Check sheet for the modelled part. Datum: model origin and axes. Units: mm. Face numbers are marked on the shaded views. A direction names the side the tool comes from. Round coordinates to 2 decimals unless told otherwise and drop trailing zeros. Loops run counter-clockwise (first coordinate to the right, second up) from the corner with the lowest first, then second, coordinate; pieces in that order, holes last. Notation, with made-up numbers: (-14.75, 67) - (20.25, 67) arc R24 ccw to (20.25, 94) - close; hole circle Ø1 at (-26, 8). An arc over 180 degrees is marked (long way). Answer in a Markdown table with one row per item. Add a question column.
(1) Cross-section at B-B on y = -45.5. Enter the section's corners in (x, z) (3 decimals).
(2) Mould release check, pull along X, two halves, no side actions. Record for the marked faces 1, 2 and 3: +X half, -X half, draft (parallel to the pull), parting line (faces both ways), or undercut.
(3) Access from +Z, -Z, +X, -X, +Y, -Y to the whole of each face (thin tool, end or side, straight path). Record for the marked faces 4, 5, 6 and 7.
(4) Cross-section at A-A on z = 7. Enter the section's corners in (x, y) (3 decimals).
(5) Thickness scan on line 1 along Z through (x, y) = (118.5, 10) (3 decimals); line 2 along Y through (x, z) = (91, 46); line 3 along X through (y, z) = (-47.5, 0.5) (3 decimals). Record the ranges inside material, lowest first.
(6) Gauge pin test, flat ends, axial feed: pin 1 (6 mm diameter, centred on y = -0.5, z = 40.5, fed in from -X); pin 2 (12 mm diameter, centred on x = 114, z = 32, fed in from +Y); pin 3 (5 mm diameter, centred on y = -18, z = 17.5, fed in from -X) (3 decimals); pin 4 (1.5 mm diameter, centred on x = 105, z = 47.5, fed in from +Y). Record the tip position at first contact, or that the pin passes through.
from build123d import *

# Parameters (mm, degrees)
F1_DEPTH = 63.5
F2_DEPTH = 25.4
F3_DEPTH = 7.9375


with BuildPart() as f1:
    # F0 (on Front) → F1 (new body, symmetric)
    with BuildSketch(Plane.XZ):
        Polygon((41.275, -9.525), (41.275, 9.525), (22.225, 9.525), (-41.275, 9.525), (-41.275, -9.525), align=None)
    extrude(amount=F1_DEPTH, both=True)

    # F0 (on Front) → F2 (join, symmetric)
    with BuildSketch(Plane.XZ):
        with BuildLine():
            Line((22.225, 9.525), (41.275, 9.525))
            Line((41.275, 9.525), (41.275, 27.5082))
            ThreePointArc((41.275, 27.5082), (45.9246798487, 38.7335201513), (57.15, 43.3832))
            Line((57.15, 43.3832), (85.725, 43.3832))
            Line((85.725, 43.3832), (89.2527830116, 43.3832))
            Line((89.2527830116, 43.3832), (89.2527830116, 62.4332))
            Line((89.2527830116, 62.4332), (57.15, 62.4332))
            add(Edge.make_bspline(
                [(49.0060559651, 61.4704113614), (51.7327824765, 61.8426488298), (54.4505405881, 62.1619414816), (57.15, 62.4332)],
                knots=[103.7473842529, 103.7473842529, 103.7473842529, 103.7473842529, 111.7441642872, 111.7441642872, 111.7441642872, 111.7441642872], degree=3))
            ThreePointArc((49.0060559651, 61.4704113614), (29.7257144996, 49.1337448438), (22.225, 27.5082))
            Line((22.225, 27.5082), (22.225, 9.525))
        make_face()
        Polygon((89.2527830116, 66.675), (89.2527830116, 62.4332), (113.3148976126, 62.4332), (114.1855414441, 43.3832), (114.427, 38.1), (140.0527830116, 38.1), (140.0527830116, 66.675), align=None)
        Polygon((89.2527830116, 62.4332), (89.2527830116, 43.3832), (114.1855414441, 43.3832), (113.3148976126, 62.4332), align=None)
        Polygon((114.1855414441, 43.3832), (89.2527830116, 43.3832), (89.2527830116, 38.1), (114.427, 38.1), align=None)
    extrude(amount=F2_DEPTH, both=True)

    # F0 (on Front) → F3 (join, symmetric)
    with BuildSketch(Plane.XZ):
        with BuildLine():
            Line((-41.275, 9.525), (22.225, 9.525))
            Line((22.225, 9.525), (22.225, 27.5082))
            ThreePointArc((22.225, 27.5082), (29.7257144996, 49.1337448438), (49.0060559651, 61.4704113614))
            add(Edge.make_bspline(
                [(-41.275, 9.525), (-23.2546272246, 42.9004266833), (13.6304745526, 56.6411346395), (49.0060559651, 61.4704113614)],
                knots=[0, 0, 0, 0, 103.7473842529, 103.7473842529, 103.7473842529, 103.7473842529], degree=3))
        make_face()
    extrude(amount=F3_DEPTH, both=True)


solid = f1.part
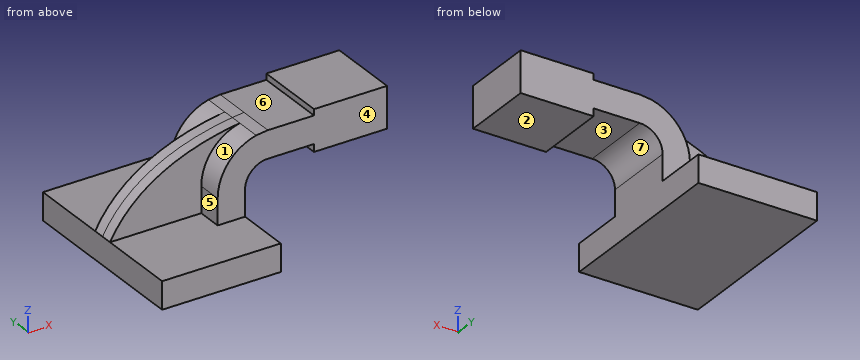
Answers:
| question | item | result |
|---|---|---|
| 1 | outline | (-41.275, -9.525) - (41.275, -9.525) - (41.275, 9.525) - (-41.275, 9.525) - close |
| 2 | face 1 | -X half |
| 2 | face 2 | draft |
| 2 | face 3 | undercut |
| 3 | face 4 | +Z, +X, -X, -Y |
| 3 | face 5 | +Z, -X, -Y |
| 3 | face 6 | +Z, -X, +Y, -Y |
| 3 | face 7 | -Z, +Y, -Y |
| 4 | outline | (-41.275, -63.5) - (41.275, -63.5) - (41.275, 63.5) - (-41.275, 63.5) - close |
| 5 | line 1 | z = 38.1 to 66.675 |
| 5 | line 2 | y = -25.4 to 25.4 |
| 5 | line 3 | x = -41.275 to 41.275 |
| 6 | pin 1 | stops at x = -16.72 |
| 6 | pin 2 | passes through |
| 6 | pin 3 | stops at x = 22.225 |
| 6 | pin 4 | stops at y = 25.4 |
